Geometry: final body of the model. Coordinates: model frame, mm. A direction names the side the tool comes from. Give positions to 0.01 mm unless a question says otherwise; leave off trailing zeros. Write each loop counter-clockwise with the first axis right and the second up, starting at its lowest first coordinate (ties: lowest second). Pieces come first, ordered by that corner, then holes. Notation, with made-up numbers: (43.25, 25) -> (75.25, 25) arc R9 cw to (75.25, 40) -> close; hole circle Ø1 at (-18, 63). An arc over 180 degrees is marked (long way). Use CSV: the item, a comma, the result in double quotes. Start each with the question number.
1) Draft query along Z for faces 1 (the face through (10, 2, -60)), 2 (the face through (19.857, -16.109, 58.752)), 3 (the face through (7.5, 2, -21)). Return one class per face: pulls with the +Z half, pulls with the -Z half, needs draft (parallel to the pull), parting line crosses it, or undercut.
2) Contact query for flat-ended pins moving along their axis: P1, Ø2, axis at x = 9, y = -7, coming from the -Z side; P2, Ø10, axis at x = -2, y = -20, coming from the -Z side; P3, Ø5.5, axis at y = 3.5, z = -21.5, coming from the +X side; P4, Ø9, axis at x = 0, z = -47.5, coming from the -Y side. Output: stop coordinate, or through.
3) Section D-D (z = 5.5). Output: boundary loops of the cut face in (x, y), plus the area to 3 significant figures.
4) Set-up query: faces 4 (the face through (12.5, 2, -4)), 5 (the face through (-6.6, 2.54, -5.86)), 6 (the face through (18.43, -5.97, 58.75)), 7 (the face through (0, -15, 51.5)). Return all of +Z, -Z, +X, -X, +Y, -Y with unobstructed straight access to the full face (end or side cutting, diameter ignored); none if empty.
5) Material intervals for line 1 (Z direction, x = -25.5, y = -16); line 2 (Z direction, x = -1.5, y = -16.5); line 3 (X direction, y = -7.5, z = 43.5), sorted ascending. Write a range as [from, to].
6) Section A-A (z = 21.5). Output: boundary loops of the cut face in (x, y), plus the area to 3 significant figures.
7) Section B-B (x = 9). Output: boundary loops of the cut face in (y, z), plus the area to 3 significant figures.
8) Section C-C (y = -14). Output: boundary loops of the cut face in (x, z).
```python
from build123d import *

# Parameters (mm, degrees)
BOSS_EXTRUDE1_DEPTH = 5
CHAMFER1_SIZE       = 5
SKETCH5_W           = 5
SKETCH5_H           = 15
BOSS_EXTRUDE3_DEPTH = 30
HOLE1_D             = 3.556
HOLE1_CBORE_D       = 6.858
HOLE1_CBORE_DEPTH   = 2.54
SKETCH9_R           = 4
CUT_EXTRUDE2_DEPTH  = 78.661122835
SKETCH10_W          = 15
SKETCH10_H          = 32.5
CUT_EXTRUDE3_DEPTH  = 78.661122835
CUT_EXTRUDE4_DEPTH  = 79.819413852
FILLET5_R           = 10
SKETCH13_W          = 15
SKETCH13_H          = 25
CUT_EXTRUDE5_DEPTH  = 78.661122835
FILLET3_R           = 3
CHAMFER3_SIZE       = 1


with BuildPart() as part:
    # Sketch1 → Boss-Extrude1 (new body)
    with BuildSketch(Plane(origin=(0, 0, 0), x_dir=(1, 0, 0), z_dir=(0, 1, 0))):
        Polygon((-12.5, 62.5), (-12.5, -57.5), (-35, -57.5), (-35, -62.5), (35, -62.5), (35, -57.5), (12.5, -57.5), (12.5, 62.5), align=None)
    extrude(amount=BOSS_EXTRUDE1_DEPTH)

    # Chamfer1
    chamfer1_edges = [part.edges().sort_by_distance(p)[0] for p in [
        (-12.5, 2.5, -62.5),
        (12.5, 2.5, -62.5),
    ]]
    chamfer(chamfer1_edges, length=CHAMFER1_SIZE)

    # Sketch5 → Boss-Extrude3 (add)
    with BuildSketch(Plane(origin=(0, 0, 0), x_dir=(-1, 0, 0), z_dir=(0, -1, 0))):
        with Locations((0, -50)):
            Rectangle(SKETCH5_W, SKETCH5_H)
        Polygon((-12.5, -57.5), (-35, -57.5), (-35, -62.5), (35, -62.5), (35, -57.5), (12.5, -57.5), (2.5, -57.5), (-2.5, -57.5), align=None)
    extrude(amount=BOSS_EXTRUDE3_DEPTH)

    # Hole1 (through all)
    with Locations(Plane(origin=(0, 0, 57.5), x_dir=(-1, 0, 0), z_dir=(0, 0, -1))):
        with Locations((-21.7, -7), (-9, -7), (9, -7), (21.7, -7), (-9, -19), (-21.7, -19), (9, -19), (21.7, -19)):
            CounterBoreHole(HOLE1_D / 2, HOLE1_CBORE_D / 2, HOLE1_CBORE_DEPTH)

    # Sketch9 → Cut-Extrude2 (cut, through all)
    with BuildSketch(Plane.XZ):
        with Locations(Location((0, -47.5, 0), (0, 0, 270))):
            Circle(SKETCH9_R)
        with Locations(Location((0, 5, 0), (0, 0, 270))):
            Circle(SKETCH9_R)
    extrude(amount=-CUT_EXTRUDE2_DEPTH, mode=Mode.SUBTRACT)

    # Sketch10 → Cut-Extrude3 (cut, through all)
    with BuildSketch(Plane.XZ):
        with Locations((0, -21.25)):
            Rectangle(SKETCH10_W, SKETCH10_H)
    extrude(amount=-CUT_EXTRUDE3_DEPTH, mode=Mode.SUBTRACT)

    # Sketch12 → Cut-Extrude4 (cut, through all)
    with BuildSketch(Plane.ZY.offset(2.5)):
        with BuildLine():
            Line((51.5, -5), (51.5, -25))
            ThreePointArc((51.5, -25), (50, -26.5), (48.5, -25))
            Line((48.5, -25), (48.5, -5))
            ThreePointArc((48.5, -5), (50, -3.5), (51.5, -5))
        make_face()
    extrude(amount=-CUT_EXTRUDE4_DEPTH, mode=Mode.SUBTRACT)

    # Fillet5
    fillet5_edges = [part.edges().sort_by_distance(p)[0] for p in [
        (-12.5, 2.5, 57.5),
        (12.5, 2.5, 57.5),
    ]]
    fillet(fillet5_edges, radius=FILLET5_R)

    # Sketch13 → Cut-Extrude5 (cut, through all)
    with BuildSketch(Plane.XZ):
        with Locations((0, 27.5)):
            Rectangle(SKETCH13_W, SKETCH13_H)
    extrude(amount=-CUT_EXTRUDE5_DEPTH, mode=Mode.SUBTRACT)

    # Fillet3
    fillet3_edges = [part.edges().sort_by_distance(p)[0] for p in [
        (7.5, 2.5, -5),
        (7.5, 2.5, -37.5),
        (-7.5, 2.5, -37.5),
        (-7.5, 2.5, -5),
        (7.5, 2.5, 40),
        (7.5, 2.5, 15),
        (-7.5, 2.5, 15),
        (-7.5, 2.5, 40),
    ]]
    fillet(fillet3_edges, radius=FILLET3_R)

    # Chamfer3
    chamfer3_edges = [part.edges().sort_by_distance(p)[0] for p in [
        (35, 5, 60),
        (-35, 5, 60),
        (0, -30, 42.5),
        (35, -30, 60),
        (-35, -30, 60),
    ]]
    chamfer(chamfer3_edges, length=CHAMFER3_SIZE)


solid = part.part
```
Answers follow:
1,face 1,"pulls with the -Z half"
1,face 2,"needs draft"
1,face 3,"undercut"
2,P1,"passes through"
2,P2,"stops at z = 42.5"
2,P3,"stops at x = 12.5"
2,P4,"stops at y = 0"
3,outline,"(-12.5, 0) -> (-3.97, 0) -> (-3.97, 5) -> (-12.5, 5) -> close; (3.97, 0) -> (12.5, 0) -> (12.5, 5) -> (3.97, 5) -> close"
3,area,"85.3 mm^2"
4,face 4,"-Z, +X, +Y, -Y"
4,face 5,"+Y, -Y"
4,face 6,"-Z"
4,face 7,"+X, -X"
5,line 1,"z = [57.5, 62.5]"
5,line 2,"z = [42.5, 48.5], [51.5, 62.5]"
5,line 3,"x = [-2.5, 2.5]"
6,outline,"(-12.5, 0) -> (-7.5, 0) -> (-7.5, 5) -> (-12.5, 5) -> close; (7.5, 0) -> (12.5, 0) -> (12.5, 5) -> (7.5, 5) -> close"
6,area,"50.0 mm^2"
7,outline,"(-30, 57.5) -> (-22.43, 57.5) -> (-22.43, 60.04) -> (-20.78, 60.04) -> (-20.78, 62.5) -> (-30, 62.5) -> close; (-17.22, 60.04) -> (-15.57, 60.04) -> (-15.57, 57.5) -> (-10.43, 57.5) -> (-10.43, 60.04) -> (-8.78, 60.04) -> (-8.78, 62.5) -> (-17.22, 62.5) -> close; (-5.22, 60.04) -> (-3.57, 60.04) -> (-3.57, 57.5) -> (0, 57.5) -> (0, -61) -> (5, -61) -> (5, 62.5) -> (-5.22, 62.5) -> close"
7,area,"715 mm^2"
8,outline,"(-35, 57.5) -> (-2.5, 57.5) -> (-2.5, 51.5) -> (2.5, 51.5) -> (2.5, 57.5) -> (35, 57.5) -> (35, 62.5) -> (-35, 62.5) -> close; (-2.5, 42.5) -> (2.5, 42.5) -> (2.5, 48.5) -> (-2.5, 48.5) -> close"
